```python
from build123d import *

# Parameters (mm, degrees)
SKETCH_1_W               = 160
SKETCH_1_H               = 80
EXTRUDE_1_DEPTH          = 15
SKETCH_2_W               = 90
SKETCH_2_H               = 50
EXTRUDE_2_DEPTH          = 45
EXTRUDE_8_DEPTH          = 30
RIB_9_REACH              = 128.886
SKETCH_7_WALL_W          = 350.771540414
SKETCH_7_WALL_H          = 10
CUT_EXTRUDE_1_DEPTH      = 35
SKETCH_10_R              = 7.5
CUT_EXTRUDE_2_DEPTH      = 127.885775405
MIRROR_3_COPY_1_SKETCH_R = 7.5
MIRROR_3_COPY_1_DEPTH    = 127.885775405
FILLET_1_R               = 12
FILLET_2_R               = 12
FILLET_3_R               = 12
FILLET_4_R               = 12
FILLET_5_R               = 15
FILLET_6_R               = 15
CUT_EXTRUDE_3_DEPTH      = 127.885775405
CUT_EXTRUDE_3_DEPTH_BACK = 127.885775405
SKETCH_11_R              = 10


with BuildPart() as part:
    # 草图1 → 凸台-拉伸1 (new body)
    with BuildSketch(Plane(origin=(0, 0, 0), x_dir=(1, 0, 0), z_dir=(0, 1, 0))):
        Rectangle(SKETCH_1_W, SKETCH_1_H)
    extrude(amount=EXTRUDE_1_DEPTH)

    # 草图2 → 凸台-拉伸2 (add)
    with BuildSketch(Plane(origin=(0, 0, 0), x_dir=(1, 0, 0), z_dir=(0, 1, 0))):
        Rectangle(SKETCH_2_W, SKETCH_2_H)
    extrude(amount=EXTRUDE_2_DEPTH)

    # 草图6 → 凸台-拉伸8 (add, symmetric)
    with BuildSketch(Plane.XY):
        with BuildLine():
            Line((0, 15), (20, 15))
            Line((20, 15), (20, 70))
            ThreePointArc((20, 70), (0, 90), (-20, 70))
            Line((-20, 70), (-20, 15))
            Line((-20, 15), (0, 15))
        make_face()
    extrude(amount=EXTRUDE_8_DEPTH, both=True)

    # 草图7 wall → 筋9 (add, up to next)
    with BuildSketch(Plane(origin=(-47.241382895, 49.396547961, 0), x_dir=(0.689655172411, 0.724137931037, 0), z_dir=(-0.724137931037, 0.689655172411, 0)), mode=Mode.PRIVATE) as rib_9_sk1:
        Rectangle(SKETCH_7_WALL_W, SKETCH_7_WALL_H)
    rib_9_tool1 = extrude(rib_9_sk1.sketch, amount=-RIB_9_REACH, mode=Mode.PRIVATE) - part.part
    rib_9 = rib_9_tool1.solids().sort_by_distance((-47.241382895, 49.396547961, 0))[0]
    add(rib_9)

    # 镜向1: 筋9 across plane
    add(rib_9.mirror(Plane(origin=(0, 0, 0), x_dir=(0, 0, 1), z_dir=(1, 0, 0))))

    # 草图8 → 切除-拉伸1 (cut)
    with BuildSketch(Plane(origin=(0, 0, 0), x_dir=(1, 0, 0), z_dir=(0, 1, 0))):
        with BuildLine():
            Line((-40, -40), (40, -40))
            Line((40, -40), (40, -35))
            ThreePointArc((40, -35), (0, 5), (-40, -35))
            Line((-40, -35), (-40, -40))
        make_face()
    extrude(amount=CUT_EXTRUDE_1_DEPTH, mode=Mode.SUBTRACT)

    # 草图10 → 切除-拉伸2 (cut, through all)
    with BuildSketch(Plane(origin=(0, 0, 0), x_dir=(1, 0, 0), z_dir=(0, 1, 0))):
        with Locations(Location((-65, 25, 0), (0, 0, 90))):
            Circle(SKETCH_10_R)
    cut_extrude_2 = extrude(amount=CUT_EXTRUDE_2_DEPTH, mode=Mode.SUBTRACT)

    # 镜向2: 切除-拉伸2 across plane
    add(cut_extrude_2.mirror(Plane(origin=(0, 0, 0), x_dir=(0, 0, 1), z_dir=(1, 0, 0))), mode=Mode.SUBTRACT)

    # 镜向3: 切除-拉伸2 across plane
    add(cut_extrude_2.mirror(Plane.XY), mode=Mode.SUBTRACT)

    # 镜向3 copy 1 sketch → 镜向3 copy 1 (cut, through all)
    with BuildSketch(Plane(origin=(0, 0, 0), x_dir=(-1, 0, 0), z_dir=(0, 1, 0))):
        with Locations(Location((-65, 25, 0), (0, 0, 90))):
            Circle(MIRROR_3_COPY_1_SKETCH_R)
    extrude(amount=MIRROR_3_COPY_1_DEPTH, mode=Mode.SUBTRACT)

    # 圆角1
    fillet_1_edges = [part.edges().sort_by_distance(p)[0] for p in [
        (-80, 7.5, -40),
    ]]
    fillet(fillet_1_edges, radius=FILLET_1_R)

    # 圆角2
    fillet_2_edges = [part.edges().sort_by_distance(p)[0] for p in [
        (80, 7.5, -40),
    ]]
    fillet(fillet_2_edges, radius=FILLET_2_R)

    # 圆角3
    fillet_3_edges = [part.edges().sort_by_distance(p)[0] for p in [
        (-80, 7.5, 40),
    ]]
    fillet(fillet_3_edges, radius=FILLET_3_R)

    # 圆角4
    fillet_4_edges = [part.edges().sort_by_distance(p)[0] for p in [
        (80, 7.5, 40),
    ]]
    fillet(fillet_4_edges, radius=FILLET_4_R)

    # 圆角5
    fillet_5_edges = [part.edges().sort_by_distance(p)[0] for p in [
        (-45, 30, -25),
    ]]
    fillet(fillet_5_edges, radius=FILLET_5_R)

    # 圆角6
    fillet_6_edges = [part.edges().sort_by_distance(p)[0] for p in [
        (45, 30, -25),
    ]]
    fillet(fillet_6_edges, radius=FILLET_6_R)

    # 草图11 → 切除-拉伸3 (cut, two sides: drawn at the far end of the back side and taken through both)
    with BuildSketch(Plane.XY.offset(-CUT_EXTRUDE_3_DEPTH_BACK)):
        with Locations((0, 70)):
            Circle(SKETCH_11_R)
    extrude(amount=CUT_EXTRUDE_3_DEPTH + CUT_EXTRUDE_3_DEPTH_BACK, mode=Mode.SUBTRACT)


solid = part.part
```
Could you check a few things on this model? Use its own coordinates, in mm. A direction names the side the tool comes from. Coordinates: 2 decimals unless noted, no trailing zeros. Order: outer loops, then holes, each group sorted by start corner. A loop starts at its lowest first (then second) coordinate and runs counter-clockwise, first axis right, second up. Notation, with made-up numbers: M -20,21 L 15,21 A33 cw 15,59 Z; hole C -35,31 d2. An arc over 180 degrees is marked long. Use a Markdown table: item, result. Add a question column.
Q1. I want a section at C-C on x = 65. List the corners of the cut face in (y, z) for me, then the cut area to 4 significant figures.
Q2. We'd pull the mould along Z, two halves only. Please class faces 6 (the cylindrical face through (70.1, 7.4, -19.5)), 7 (the flat face through (45, 30, -7)), 8 (the cylindrical face through (-40.72, 30.21, -20.49)): pulls with the +Z half, pulls with the -Z half, needs draft (parallel to the pull), parting line crosses it, or undercut.
Q3. I want a section at D-D on y = 63. List the corners of the cut face in (x, z) for me.
Q4. I want a section at A-A on x = 0. List the corners of the cut face in (y, z) for me, then the cut area to 4 significant figures.
Q5. I'm going to push flat-ended pins straight in: pin 1 (12.5 mm diameter, centred on x = -28.5, y = 34, fed in from +Z); pin 2 (23 mm diameter, centred on x = 0, y = 70, fed in from -Z); pin 3 (20 mm diameter, centred on y = 50.5, z = 12, fed in from -X). Where does each tip first touch, or does it pass through?
Q6. Which directions (+Z, -Z, +X, -X, +Y, -Y) give clear straight access to the entire face, cutting with the end or side of a thin tool? Please do faces 1 (the cylindrical face through (0.88, 17.26, -4.99)), 2 (the flat face through (-45, 30, -7)), 3 (the flat face through (0, 45, -30)), 4 (the flat face through (-45, 30, 15)), 5 (the flat face through (25, 30, -25)).
Q7. If I drill on L1, parallel to Z at x = -65, y = 9.75; L2, parallel to X at y = 5, z = 25; L3, parallel to X at y = 8.5, z = -22.5, over which ranges is the centre line in solid material (lowest first)?
Q8. I want a section at B-B on z = -3. List the corners of the cut face in (x, y) for me.
Checked values:
| question | item | result |
|---|---|---|
| 1 | outline | M 0,-40 L 15,-40 L 15,-32.5 L 0,-32.5 Z; M 0,-17.5 L 15,-17.5 L 15,-5 L 30.75,-5 L 30.75,5 L 15,5 L 15,17.5 L 0,17.5 Z; M 0,32.5 L 15,32.5 L 15,40 L 0,40 Z |
| 1 | area | 907.5 mm² |
| 2 | face 6 | undercut |
| 2 | face 7 | needs draft |
| 2 | face 8 | pulls with the -Z half |
| 3 | outline | M -34.29,-5 L -20,-5 L -20,-30 L -7.14,-30 L -7.14,30 L -20,30 L -20,5 L -34.29,5 Z; M 7.14,-30 L 20,-30 L 20,-5 L 34.29,-5 L 34.29,5 L 20,5 L 20,30 L 7.14,30 Z |
| 4 | outline | M 0,-40 L 15,-40 L 15,-30 L 60,-30 L 60,30 L 35,30 L 35,-5 L 0,-5 Z; M 80,-30 L 90,-30 L 90,30 L 80,30 Z |
| 4 | area | 3,125 mm² |
| 5 | pin 1 | z = 25 |
| 5 | pin 2 | z = -30 |
| 5 | pin 3 | x = -52.99 |
| 6 | face 1 | +Z, -Y |
| 6 | face 2 | -Z, -X, +Y |
| 6 | face 3 | -Z, +X, -X, +Y |
| 6 | face 4 | +Z, -X, +Y |
| 6 | face 5 | -Z, +X, +Y |
| 7 | L1 | -40 to -32.5, -17.5 to 17.5, 32.5 to 40 |
| 7 | L2 | -80 to -72.5, -57.5 to -38.73, 38.73 to 57.5, 72.5 to 80 |
| 7 | L3 | -80 to -72.07, -57.93 to 57.93, 72.07 to 80 |
| 8 | outline | M -80,0 L -12.49,0 L -12.49,35 L 12.49,35 L 12.49,0 L 80,0 L 80,15 L 14.48,83.79 A20 ccw -14.48,83.79 L -80,15 Z; hole C 0,70 d20 |
